The model under review builds one solid part; all positions refer to its coordinate system, in mm. Give positions to 0.01 mm unless a question says otherwise; leave off trailing zeros. Order: outer loops, then holes, each group sorted by start corner. A loop starts at its lowest first (then second) coordinate and runs counter-clockwise, first axis right, second up. Notation, with made-up numbers: M 64.25,26.25 L 70.25,26.25 A24 cw 70.25,40.25 Z; hole C 27,-35.5 d3. An arc over 180 degrees is marked long. One line per question, with ' | ' between items. Start each with the question number.
1. We need section B-B on x = 25. Write out the cut boundary in (y, z), then the cut area to 3 significant figures.
2. Wall thickness on L1, parallel to X at y = 4.5, z = 1.5; L2, parallel to Y at x = 27.5, z = 3; L3, parallel to X at y = 9.5, z = 8.5: over which ranges is each line inside the solid? List them lowest first.
3. The part is to be moulded in two halves that separate along X. For faces 1 (the face through (11, 12, 10)), 2 (the face through (21.49, 8.46, 5.18)), 3 (the face through (23.6, 8.946, 5.171)), 4 (the face through (0, 10, 5)), say which applies: +X half, -X half, draft (parallel to the pull), parting line (faces both ways), or undercut.
4. Insertion check: P1, Ø10, axis at x = 16, y = 9, coming from the -Z side; P2, Ø1.5, axis at y = 2.5, z = 6.5, coming from the +X side. Each pin has a flat end and moves straight along its axis. Give the tip position at first contact, or say it passes through.
5. We need section A-A on y = 2.25. Write out the cut boundary in (x, z), then the cut area to 3 significant figures.
Autodesk Inventor part; units mm, degrees
ref_plane "Work Plane1" through (18, 0, 0) normal (-0.7071068, 0.7071068, 0) x (0, 0, 1)
ref_plane "YZ Plane" through (0, 0, 0) normal (1, 0, 0) x (0, 1, 0)
ref_plane "XZ Plane" through (0, 0, 0) normal (0, 1, 0) x (-1, 0, 0)
sketch "Sketch1" plane through (0, 0, 0) normal (0, 0, 1) x (1, 0, 0)
  line L0 (0, 0) -> (18, 0)
  line L1 (30, 12) -> (30, 20)
  line L2 (30, 20) -> (0, 20)
  line L3 (0, 20) -> (0, 0)
  arc A0 (30, 12) -> (18, 0) centre (30, 0) ccw
  dimension "d0" = 30
  dimension "d1" = 20
  dimension "d2" = 12
extrude "Extrusion1" add sketch "Sketch1" along normal blind 10
sketch "Sketch2" plane through (0, 0, 0) normal (0, -1, 0) x (1, 0, 0)
  line L0 (6.7288, 8.7537) -> (12.1656, 8.7537) construction
  line L1 (12.1656, 8.7537) -> (12.1656, 1.727) construction
  line L2 (12.1656, 1.727) -> (6.7288, 1.727) construction
  line L3 (6.7288, 1.727) -> (6.7288, 8.7537) construction
sketch "Sketch3" plane through (30, 12, 0) normal (1, 0, 0) x (0, 0, -1)
  line L0 (-8.6261, 1.3146) -> (-8.6261, 6.7514) construction
  line L1 (-8.6261, 6.7514) -> (-1.482, 6.7514) construction
  line L2 (-1.482, 6.7514) -> (-1.482, 1.3146) construction
  line L3 (-1.482, 1.3146) -> (-8.6261, 1.3146) construction
sketch "Sketch4" plane through (0, 20, 0) normal (0, 1, 0) x (1, 0, 0)
  line L0 (16.9923, -8.3919) -> (11.5555, -8.3919) construction
  line L1 (11.5555, -8.3919) -> (11.5555, -1.3919) construction
  line L2 (11.5555, -1.3919) -> (16.9923, -1.3919) construction
  line L3 (16.9923, -1.3919) -> (16.9923, -8.3919) construction
sketch "Sketch5" plane through (0, 0, 0) normal (-1, 0, 0) x (0, 0, 1)
  line L0 (8.5269, 13.0876) -> (8.5269, 7.6509) construction
  line L1 (8.5269, 7.6509) -> (1.5002, 7.6509) construction
  line L2 (1.5002, 7.6509) -> (1.5002, 13.0876) construction
  line L3 (1.5002, 13.0876) -> (8.5269, 13.0876) construction
sketch "Sketch6" plane through (0, 0, 10) normal (0, 0, 1) x (1, 0, 0)
  line L0 (8.4775, 14.4017) -> (13.9142, 14.4017) construction
  line L1 (13.9142, 14.4017) -> (13.9142, 7.4924) construction
  line L2 (13.9142, 7.4924) -> (8.4775, 7.4924) construction
  line L3 (8.4775, 7.4924) -> (8.4775, 14.4017) construction
sketch "Sketch7" plane through (0, 0, 0) normal (0, 0, -1) x (-1, 0, 0)
  line L0 (-16.3171, 15.4982) -> (-10.8803, 15.4982) construction
  line L1 (-10.8803, 15.4982) -> (-10.8803, 8.3541) construction
  line L2 (-10.8803, 8.3541) -> (-16.3171, 8.3541) construction
  line L3 (-16.3171, 8.3541) -> (-16.3171, 15.4982) construction
ref_plane "Work Plane1" through (18, 0, 0) normal (-0.7071068, 0.7071068, 0) x (0, 0, 1)
sketch "Sketch9" plane through (18, 0, 0) normal (-0.7071068, 0.7071068, 0) x (0, 0, 1)
  line L0 (8.7931, 11.1492) -> (8.7931, 5.7124) construction
  line L1 (8.7931, 5.7124) -> (1.7665, 5.7124) construction
  line L2 (1.7665, 5.7124) -> (1.7665, 11.1492) construction
  line L3 (1.7665, 11.1492) -> (8.7931, 11.1492) construction
  spline S0 degree 4 poles (5.2185, 10.7437) (6.4616, 10.7437) (7.9768, 10.2315) (8.7931, 9.2284) (8.7931, 8.4601) knots 0 0 0 0 0 1 1 1 1 1
  spline S1 degree 5 poles (8.7931, 8.4601) (8.7931, 7.8999) (8.3396, 7.0463) (7.486, 6.4967) (6.2589, 6.1819) (5.2185, 6.1819) knots 0 0 0 0 0 0 1 1 1 1 1 1
  spline S2 degree 4 poles (5.2185, 6.1819) (3.986, 6.1819) (2.4707, 6.6888) (1.6491, 7.6972) (1.6491, 8.4601) knots 0 0 0 0 0 1 1 1 1 1
  spline S3 degree 2 poles (1.6491, 8.4601) (1.6491, 9.4739) (2.3694, 10.0501) knots 0 0 0 1 1 1
  spline S4 degree 2 poles (2.3694, 10.0501) (3.2497, 10.7437) (5.2185, 10.7437) knots 0 0 0 1 1 1
  spline S5 degree 3 poles (5.2185, 9.858) (3.4898, 9.858) (2.3534, 9.0524) (2.3534, 8.4601) knots 0 0 0 0 1 1 1 1
  spline S6 degree 3 poles (2.3534, 8.4601) (2.3534, 7.8733) (3.4951, 7.0676) (5.2185, 7.0676) knots 0 0 0 0 1 1 1 1
  spline S7 degree 3 poles (5.2185, 7.0676) (6.9471, 7.0676) (8.0835, 7.8733) (8.0835, 8.4708) knots 0 0 0 0 1 1 1 1
  spline S8 degree 2 poles (8.0835, 8.4708) (8.0835, 9.063) (7.582, 9.4152) knots 0 0 0 1 1 1
  spline S9 degree 2 poles (7.582, 9.4152) (6.9418, 9.858) (5.2185, 9.858) knots 0 0 0 1 1 1
emboss "Emboss1" sketch "Sketch9" operation add depth 1 direction (0.7071068, -0.7071068, 0) wrap yes faces at (21.8379, 8.7966, 6.6667)
properties part number "block"
Entries:
1) outline: M 10.91,0 L 20,0 L 20,10 L 10.91,10 Z | area: 90.9 mm^2
2) L1: x = 0 to 18.88 | L2: y = 11.74 to 20 | L3: x = 0 to 22.67
3) face 1: draft | face 2: undercut | face 3: +X half | face 4: -X half
4) P1: stops at z = 0 | P2: stops at x = 18.45
5) outline: M 0,0 L 18.21,0 L 18.21,10 L 0,10 Z | area: 182 mm^2
